The model under review builds one solid part; all positions refer to its coordinate system, in mm. A direction names the side the tool comes from. Coordinates: 2 decimals unless noted, no trailing zeros. Write each loop counter-clockwise with the first axis right and the second up, starting at its lowest first coordinate (ties: lowest second). Pieces come first, ordered by that corner, then holes.
1) For line 1 (X direction, y = -1.5, z = -85); line 2 (Z direction, x = -7.25, y = 2.75); line 3 (X direction, y = 0.25, z = -83), list the stretches that pass through material, from the lowest coordinate up.
2) Machinability: for faces 4 (the cylindrical face through (-0.17, 2.22, -84.93)), 5 (the flat face through (0, 0, -90)), which of the approach directions +Z, -Z, +X, -X, +Y, -Y give a long, thin tool a straight path to every point of the face, cutting with its end or side? Answer none if there is none.
3) For P1, Ø1, axis at x = 0, z = -9.5, coming from the -Y side; P2, Ø5, axis at x = 5.5, z = -37, coming from the +Y side; P3, Ø1, axis at y = 5, z = -37.5, coming from the +X side, all flat-tipped, find the tip position at first contact; note any pin that passes through.
4) Add section B-B, the plane y = -3.25. State the section outline as (x, z) points.
5) Mouldability with a two-part tool opening along Y and no side actions: class faces 1 (the cylindrical face through (-1.973, -8.884, -1.479)), 2 (the cylindrical face through (2.97, -2.21, -84.93)), 3 (the flat face through (-1, -7, -3)) as released by +Y, released by -Y, zero draft, split by the parting line, or undercut.
6) Add section C-C, the plane z = -65.5. State the section outline as (x, y) points, then the cut area to 3 significant figures.
7) Add section A-A, the plane x = 5.5. State the section outline as (y, z) points.
from build123d import *

# Parameters (mm, degrees)
ESBO_O1_R                 = 9.1
RESSALTO_EXTRUS_O1_DEPTH  = 3
ESBO_O2_R                 = 6.7
RESSALTO_EXTRUS_O2_DEPTH  = 87
FURO_ROSCADO_DE_M21_D     = 1.6
FURO_ROSCADO_DE_M21_DEPTH = 10
FURO_ROSCADO_DE_M21_TIP   = 0.480688495


with BuildPart() as part:
    # Esboço1 → Ressalto-extrusão1 (new body)
    with BuildSketch(Plane.XY):
        Circle(ESBO_O1_R)
    extrude(amount=-RESSALTO_EXTRUS_O1_DEPTH)

    # Esboço2 → Ressalto-extrusão2 (add)
    with BuildSketch(Plane(origin=(0, 0, -3), x_dir=(-1, 0, 0), z_dir=(0, 0, -1))):
        Circle(ESBO_O2_R)
    extrude(amount=RESSALTO_EXTRUS_O2_DEPTH)

    # Furo roscado de M21
    with Locations(Plane(origin=(0, 0, -90), x_dir=(-1, 0, 0), z_dir=(0, 0, -1))):
        with Locations((-2.598076211, -1.5), (0, 3), (2.598076211, -1.5)):
            Hole(FURO_ROSCADO_DE_M21_D / 2, depth=FURO_ROSCADO_DE_M21_DEPTH)
            with Locations((0, 0, -(FURO_ROSCADO_DE_M21_DEPTH + FURO_ROSCADO_DE_M21_TIP / 2))):  # 118° drill point
                Cone(0, FURO_ROSCADO_DE_M21_D / 2, FURO_ROSCADO_DE_M21_TIP, mode=Mode.SUBTRACT)


solid = part.part
Geometry results:
1. line 1: x = -6.53 to -3.4, -1.8 to 1.8, 3.4 to 6.53
1. line 2: z = -3 to 0
1. line 3: x = -6.7 to 6.7
2. face 4: -Z
2. face 5: -Z, +X, -X, +Y, -Y
3. P1: stops at y = -6.7
3. P2: stops at y = 5.99
3. P3: stops at x = 4.96
4. outline: (-8.5, -3) - (-5.86, -3) - (-5.86, -90) - (5.86, -90) - (5.86, -3) - (8.5, -3) - (8.5, 0) - (-8.5, 0) - close
5. face 1: split by the parting line
5. face 2: undercut
5. face 3: zero draft
6. outline: circle Ø13.4 at (0, 0)
6. area: 141 mm2
7. outline: (-7.25, -3) - (-3.83, -3) - (-3.83, -90) - (3.83, -90) - (3.83, -3) - (7.25, -3) - (7.25, 0) - (-7.25, 0) - close
